Answer from the drawing. Dimensions are ordinates in mm from the lowest x, y and z of the part. A direction names the side the tool comes from. Round coordinates to 2 decimals unless told otherwise and drop trailing zeros. Order: outer loops, then holes, each group sorted by start corner. A loop starts at its lowest first (then second) coordinate and runs counter-clockwise, first axis right, second up. Notation, with made-up numbers: M -24.75,0.25 L -16.75,0.25 A18 cw -16.75,33.25 Z; hole C 8,-2 d3. An arc over 180 degrees is marked long. Write item = value, one per line. Start each with the question number.
(1) A cutting plane is placed at C-C, the plane z = 18.45. Determine the outline of the cut face in (x, y), and give its area (3 significant figures).
(2) A cutting plane is placed at A-A, the plane y = 8.55. Determine the outline of the cut face in (x, z).
(3) Straight lines are drawn through the part: probe 1 along Y at (x, z) = (12, 53.4); probe 2 along Y at (x, z) = (46.25, 18.45); probe 3 along X at (y, z) = (21.75, 7.5). For each, find the intervals that lie inside material, in ascending order. Write a range as from..to.
(4) For a pull along X with two mould halves and no side action, classify the marked faces 1, 2 and 3 as released by +X, released by -X, zero draft, split by the parting line, or undercut.
(5) Each of these flat-tipped pins is pushed along its axis until it touches: pin 1 (10 mm diameter, centred on y = 13, z = 6.5, fed in from -X); pin 2 (22.5 mm diameter, centred on x = 18.5, z = 36, fed in from +Y); pin 3 (1.5 mm diameter, centred on y = 13, z = 20, fed in from -X); pin 4 (3.5 mm diameter, centred on y = 13.55, z = 18.45, fed in from -X). Where does it stop, or does it pass through?
(6) A cutting plane is placed at B-B, the plane z = 53.4. Determine the outline of the cut face in (x, y), and give its area (3 significant figures).
(7) Which of the six approach directions +Z, -Z, +X, -X, +Y, -Y give full straight-line access (tool end or side, diameter ignored) to the marked faces 4 and 5?
(8) A cutting plane is placed at D-D, the plane y = 12.5. Determine the outline of the cut face in (x, z).
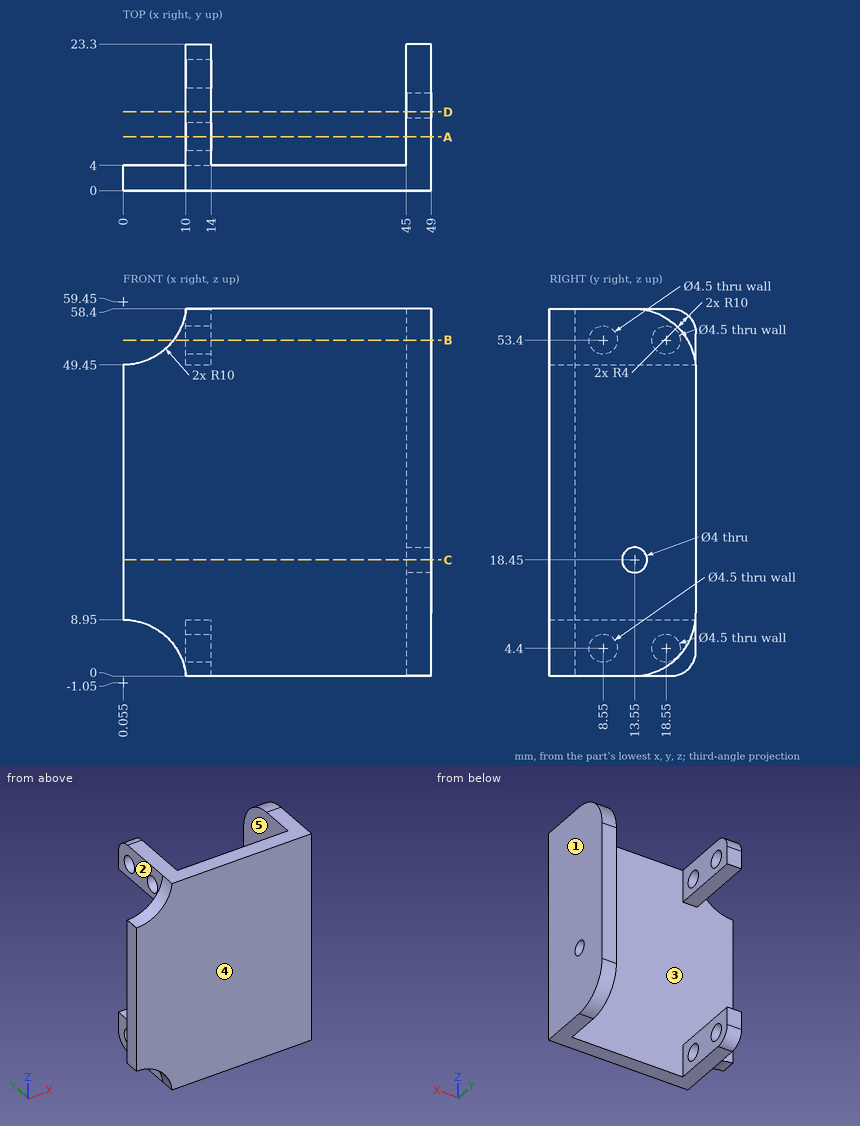
Reported:
q1.outline = M 0,0 L 49,0 L 49,11.55 L 45,11.55 L 45,4 L 0,4 Z; M 45,15.55 L 49,15.55 L 49,23.3 L 45,23.3 Z
q1.area = 257 mm²
q2.outline = M 10,0 L 14,0 L 14,2.15 L 10,2.15 Z; M 10,6.65 L 14,6.65 L 14,8.95 L 10,8.95 Z; M 10,49.45 L 14,49.45 L 14,51.15 L 10,51.15 Z; M 10,55.65 L 14,55.65 L 14,58.4 L 10,58.4 Z; M 45,0 L 49,0 L 49,58.4 L 45,58.4 Z
q3.probe_1 = 0..6.3, 10.8..16.3, 20.8..23.3
q3.probe_2 = 0..11.55, 15.55..23.3
q3.probe_3 = 10..14, 45..49
q4.face_1 = released by +X
q4.face_2 = released by -X
q4.face_3 = undercut
q5.pin_1 = 10
q5.pin_2 = 4
q5.pin_3 = 45
q5.pin_4 = through
q6.outline = M 8.02,0 L 49,0 L 49,21.96 L 45,21.96 L 45,4 L 14,4 L 14,6.3 L 10,6.3 L 10,4 L 8.02,4 Z; M 10,10.8 L 14,10.8 L 14,16.3 L 10,16.3 Z; M 10,20.8 L 14,20.8 L 14,23.3 L 10,23.3 Z
q6.area = 277 mm²
q7.face_4 = +Z, -Z, +X, -X, -Y
q7.face_5 = +Z, -Z, +Y
q8.outline = M 10,0 L 14,0 L 14,8.95 L 10,8.95 Z; M 10,49.45 L 14,49.45 L 14,58.4 L 10,58.4 Z; M 45,0 L 49,0 L 49,16.75 L 45,16.75 Z; M 45,20.15 L 49,20.15 L 49,58.4 L 45,58.4 Z
